from build123d import *

# Parameters (mm, degrees)
F1_DEPTH        = 8
F1_DEPTH_BACK   = 6
F2_R            = 8.3
F2_R_2          = 2.95
F3_DEPTH        = 3
F3_DEPTH_BACK   = 3
F5_DEPTH        = 3.3
F5_DEPTH_BACK   = 3.3
F7_START        = -14
F6_R            = 3.15
F7_DEPTH        = 26
F9_DEPTH        = 5
F10_W           = 15
F10_H           = 2.9
F11_DEPTH       = 6.4
F12_W           = 1
F12_H           = 6.5
F13_DEPTH       = 3.5
F14_T4_DEPTH    = 31.8168298797
F16_D           = 3.2
F16_DEPTH       = 11
F16_CBORE_D     = 6.5
F16_CBORE_DEPTH = 2.5
F16_TIP         = 0.9613769904
F18_D           = 3.2
F18_CBORE_D     = 6.2
F18_CBORE_DEPTH = 2.6
F20_DEPTH       = 25
F20_DEPTH_BACK  = 25
F21_W           = 5.7
F21_H           = 2.5
F22_DEPTH       = 25
F22_DEPTH_BACK  = 25


# Not quite as in the source:
# - a fillet or chamfer that OpenCascade refuses, or shapes differently, is made with other operations: its cross-section is extruded or revolved along the edge and cut away or added


with BuildPart() as f1:
    # F0 (on Top) → F1 (new body, two sides)
    with BuildSketch(Plane.XY) as f1_sk:
        with BuildLine():
            Line((-21, -8.5), (1.608228737, -5.0218109635))
            ThreePointArc((1.608228737, -5.0218109635), (4.0358618997, -3.6728476468), (5, -1.0683241729))
            Line((5, -1.0683241729), (5, 1.0683241729))
            ThreePointArc((5, 1.0683241729), (4.0358618997, 3.6728476468), (1.608228737, 5.0218109635))
            Line((1.608228737, 5.0218109635), (-21, 8.5))
            Line((-21, 8.5), (-21, -8.5))
        make_face()
    extrude(amount=F1_DEPTH)
    extrude(f1_sk.sketch, amount=-F1_DEPTH_BACK)

    # F2 (on Top) → F3 (cut, two sides)
    with BuildSketch(Plane.XY) as f3_sk:
        Circle(F2_R)
        Circle(F2_R_2, mode=Mode.SUBTRACT)
    extrude(amount=-F3_DEPTH, mode=Mode.SUBTRACT)
    extrude(f3_sk.sketch, amount=F3_DEPTH_BACK, mode=Mode.SUBTRACT)

    # F4 (on Top) → F5 (cut, two sides)
    with BuildSketch(Plane.XY) as f5_sk:
        with BuildLine():
            ThreePointArc((5, -2.1685248442), (-5.45, 0), (5, 2.1685248442))
            Line((5, 2.1685248442), (5, 8.3120394609))
            ThreePointArc((5, 8.3120394609), (-9.7, 0), (5, -8.3120394609))
            Line((5, -8.3120394609), (5, -2.1685248442))
        make_face()
    extrude(amount=F5_DEPTH, mode=Mode.SUBTRACT)
    extrude(f5_sk.sketch, amount=-F5_DEPTH_BACK, mode=Mode.SUBTRACT)

    # F6 (on Right) → F7 (cut)
    with BuildSketch(Plane.YZ.offset(F7_START)):
        with Locations((0, 0.5)):
            Circle(F6_R)
    extrude(amount=-F7_DEPTH, mode=Mode.SUBTRACT)

    # F8 (on face) → F9 (cut)
    with BuildSketch(Plane(origin=(-21, 0, 0), x_dir=(0, -1, 0), z_dir=(-1, 0, 0))):
        Polygon((2.9444863729, 5.6), (-2.9444863729, 5.6), (-5.8889727457, 0.5), (-2.9444863729, -4.6), (2.9444863729, -4.6), (5.8889727457, 0.5), align=None)
    extrude(amount=-F9_DEPTH, mode=Mode.SUBTRACT)

    # F10 (on face) → F11 (join)
    with BuildSketch(Plane.XY.offset(8)):
        with Locations((-13.5, 4.5)):
            Rectangle(F10_W, F10_H)
        with Locations((-13.5, -4.5)):
            Rectangle(F10_W, F10_H)
    extrude(amount=F11_DEPTH)

    # F12 (on face) → F13 (join)
    with BuildSketch(Plane.XY.offset(8)):
        with Locations((-6.5, 0)):
            Rectangle(F12_W, F12_H)
    extrude(amount=F13_DEPTH)

    # F14: chamfer of 5 on 1 edges, made by hand


with BuildPart() as f14_tool2:
    # F14_s3 → F14_t4 (new body)
    with BuildSketch(Plane.XZ.offset(-15.9084149398)):
        Polygon((-7, 13), (-12, 8), (-7, 8), align=None)
    extrude(amount=F14_T4_DEPTH)

    split(bisect_by=Plane.XY.offset(11.5), keep=Keep.BOTTOM)

    split(bisect_by=Plane.XZ.offset(-5.95), keep=Keep.TOP)

    split(bisect_by=Plane.XZ.offset(5.95), keep=Keep.BOTTOM)


with BuildPart() as f1_1:
    add(f1.part)

    # F14_t1: union F14_tool2
    add(f14_tool2.part)

    # F16
    with Locations(Plane(origin=(0, 0, -6), x_dir=(1, 0, 0), z_dir=(0, 0, -1))):
        with Locations((-11, -4.5), (-11, 4.5)):
            CounterBoreHole(F16_D / 2, F16_CBORE_D / 2, F16_CBORE_DEPTH, depth=F16_DEPTH)
            with Locations((0, 0, -(F16_DEPTH + F16_TIP / 2))):  # 118° drill point
                Cone(0, F16_D / 2, F16_TIP, mode=Mode.SUBTRACT)

    # F18 (through all)
    with Locations(Plane(origin=(0, 0, -6), x_dir=(1, 0, 0), z_dir=(0, 0, -1))):
        with Locations((0, 0)):
            CounterBoreHole(F18_D / 2, F18_CBORE_D / 2, F18_CBORE_DEPTH)

    # F19 (on Front) → F20 (cut, two sides)
    with BuildSketch(Plane.XZ) as f20_sk:
        Polygon((9.8263500258, -7.5822613659), (9.9938229204, 3), (-6.1094067059, 3), (-6.1094067059, -2.3), (-14.3, -2.3), (-14.3, -7.5822613659), align=None)
    extrude(amount=-F20_DEPTH, mode=Mode.SUBTRACT)
    extrude(f20_sk.sketch, amount=F20_DEPTH_BACK, mode=Mode.SUBTRACT)

    # F21 (on Front) → F22 (cut, two sides)
    with BuildSketch(Plane.XZ) as f22_sk:
        with Locations((-11, 5)):
            Rectangle(F21_W, F21_H)
    extrude(amount=-F22_DEPTH, mode=Mode.SUBTRACT)
    extrude(f22_sk.sketch, amount=F22_DEPTH_BACK, mode=Mode.SUBTRACT)


solid = f1_1.part
Geometry check sheet. Reference: the model listing, model coordinates, mm. A direction names the side the tool comes from. Give positions to 0.01 mm unless a question says otherwise; leave off trailing zeros. Loops run counter-clockwise (first coordinate to the right, second up) from the corner with the lowest first, then second, coordinate; pieces in that order, holes last. Notation, with made-up numbers: (68.5, 16) -> (123.5, 16) arc R17 cw to (123.5, 35) -> close; hole circle Ø3 at (20.5, 14). An arc over 180 degrees is marked (long way). Answer in a Markdown table with one row per item. Add a question column.
1) Cross-section at D-D on x = 0. Record the boundary of the cut face in (y, z), and give its area (3 significant figures).
2) Material ranges on probe 1 along Y at (x, z) = (-11, 1); probe 2 along Z at (x, y) = (-15.4, 0); probe 3 along Y at (x, z) = (-19.75, 11.5), recorded low to high. Write a range as from..to.
3) Cross-section at A-A on y = 0.75. State how many separate pieces and enclosed holes the cut face has, and give its area (3 significant figures).
4) Draft check along Z on faces 1 (the face through (-7, 0, 11.5)), 2 (the face through (4.062, 3.643, 5.535)), 3 (the face through (-14, 0, 1)). Enter one of: pulls with the +Z half, pulls with the -Z half, needs draft (parallel to the pull), parting line crosses it, or undercut.
5) Cross-section at B-B on z = 1.75. Record the boundary of the cut face in (x, y), and give its area (3 significant figures).
6) Gauge pin test, flat ends, axial feed: P1, Ø3, axis at x = -13, z = 1.5, coming from the -Y side; P2, Ø4, axis at y = 3.5, z = -4.5, coming from the +X side; P3, Ø6, axis at x = -6.5, y = -3, coming from the -Z side; P4, Ø1, axis at x = -4, y = 7, coming from the -Z side. Record the tip position at first contact, or that the pin passes through.
7) Cross-section at C-C on x = -11. Record the boundary of the cut face in (y, z).
8) Set-up check for faces 4 (the face through (-8.15, 0, 5)), 5 (the face through (-12, 0, -2.3)), 6 (the face through (-19, 0, -4.6)), 7 (the face through (-15, 3.05, 11)): record each of +Z, -Z, +X, -X, +Y, -Y from which the full face is reachable in a straight line by a thin tool's end or side.
Outcome:
| question | item | result |
|---|---|---|
| 1 | outline | (-5.27, 3) -> (-1.6, 3) -> (-1.6, 8) -> (-5.27, 8) -> close; (1.6, 3) -> (5.27, 3) -> (5.27, 8) -> (1.6, 8) -> close |
| 1 | area | 36.7 mm^2 |
| 2 | probe 1 | y = -6.96..-6.1, -2.9..2.9, 6.1..6.96 |
| 2 | probe 2 | z = -6..-2.65, 3.65..8 |
| 2 | probe 3 | y = -5.95..-3.05, 3.05..5.95 |
| 3 | separate pieces | 3 |
| 3 | enclosed holes | 1 |
| 3 | area | 137 mm^2 |
| 4 | face 1 | pulls with the +Z half |
| 4 | face 2 | needs draft |
| 4 | face 3 | undercut |
| 5 | outline | (-21, -8.5) -> (-7.3, -6.39) arc R9.7 cw to (-7.3, 6.39) -> (-21, 8.5) -> (-21, 5.17) -> (-16, 5.17) -> (-16, 2.89) -> (-14, 2.89) -> (-14, -2.89) -> (-16, -2.89) -> (-16, -5.17) -> (-21, -5.17) -> close; hole circle Ø3.2 at (-11, -4.5); hole circle Ø3.2 at (-11, 4.5) |
| 5 | area | 104 mm^2 |
| 6 | P1 | stops at y = -7.5 |
| 6 | P2 | stops at x = -14.3 |
| 6 | P3 | stops at z = -2.3 |
| 6 | P4 | passes through |
| 7 | outline | (-6.96, -2.3) -> (-6.1, -2.3) -> (-6.1, 3.75) -> (-6.96, 3.75) -> close; (-6.96, 6.25) -> (6.96, 6.25) -> (6.96, 8) -> (5.95, 8) -> (5.95, 14.4) -> (3.05, 14.4) -> (3.05, 9) -> (-3.05, 9) -> (-3.05, 14.4) -> (-5.95, 14.4) -> (-5.95, 8) -> (-6.96, 8) -> close; (-2.9, -2.3) -> (2.9, -2.3) -> (2.9, 3.75) -> (-2.9, 3.75) -> close; (6.1, -2.3) -> (6.96, -2.3) -> (6.96, 3.75) -> (6.1, 3.75) -> close |
| 8 | face 4 | +Y, -Y |
| 8 | face 5 | -Z, +X, +Y, -Y |
| 8 | face 6 | -X |
| 8 | face 7 | +Z, -X |
